Verification items for the finished model (mm, model axes). Face numbers are marked on the shaded views. Give positions to 0.01 mm unless a question says otherwise; leave off trailing zeros. Write each loop counter-clockwise with the first axis right and the second up, starting at its lowest first coordinate (ties: lowest second). Pieces come first, ordered by that corner, then holes.
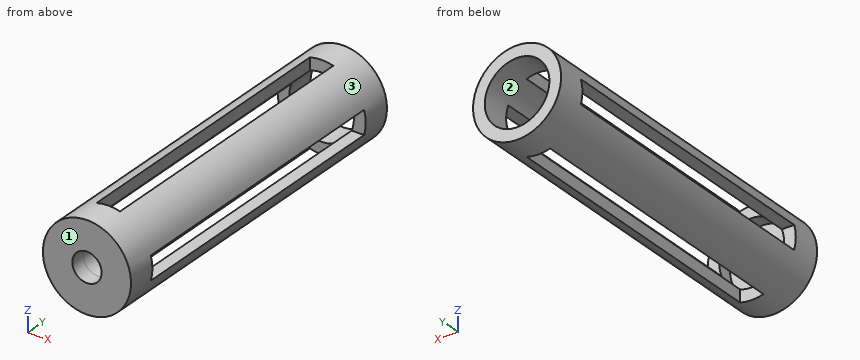
from build123d import *

# Parameters (mm, degrees)
SKETCH1_R               = 19.05
SKETCH1_R_2             = 13.97
BOSS_EXTRUDE1_DEPTH     = 152.4
SKETCH2_R               = 13.97
BOSS_EXTRUDE2_DEPTH     = 6.35
SKETCH3_R               = 2.2479
CUT_EXTRUDE1_DEPTH      = 3.54
CUT_EXTRUDE1_DEPTH_BACK = 36.56
SKETCH5_W               = 10.16
SKETCH5_H               = 127
CUT_EXTRUDE5_DEPTH      = 20.0500001
CUT_EXTRUDE5_DEPTH_BACK = 20.0500001
SKETCH8_W               = 10.16
SKETCH8_H               = 127
CUT_EXTRUDE6_DEPTH      = 20.050000101
CUT_EXTRUDE6_DEPTH_BACK = 20.050000101
SKETCH7_R               = 6.35
CUT_EXTRUDE4_DEPTH      = 7.35
SKETCH9_R               = 8.89
SKETCH9_R_2             = 6.35
BOSS_EXTRUDE3_DEPTH     = 19.05
SKETCH10_R              = 8.89
SKETCH10_R_2            = 5.08
BOSS_EXTRUDE4_DEPTH     = 5.08


with BuildPart() as part:
    # Sketch1 → Boss-Extrude1 (new body)
    with BuildSketch(Plane(origin=(0, 0, 0), x_dir=(1, 0, 0), z_dir=(0, 1, 0))):
        Circle(SKETCH1_R)
        Circle(SKETCH1_R_2, mode=Mode.SUBTRACT)
    extrude(amount=BOSS_EXTRUDE1_DEPTH)

    # Sketch2 → Boss-Extrude2 (add)
    with BuildSketch(Plane.XZ):
        Circle(SKETCH2_R)
    extrude(amount=-BOSS_EXTRUDE2_DEPTH)

    # Sketch3 → Cut-Extrude1 (cut, two sides)
    with BuildSketch(Plane.XY.offset(16.51)) as cut_extrude1_sk:
        with Locations((0, 101.6)):
            Circle(SKETCH3_R)
    extrude(amount=CUT_EXTRUDE1_DEPTH, mode=Mode.SUBTRACT)
    extrude(cut_extrude1_sk.sketch, amount=-CUT_EXTRUDE1_DEPTH_BACK, mode=Mode.SUBTRACT)

    # Sketch5 → Cut-Extrude5 (cut, two sides)
    with BuildSketch(Plane(origin=(0, 0, 0), x_dir=(0, 0, -1), z_dir=(1, 0, 0))) as cut_extrude5_sk:
        with Locations((0, 76.2)):
            Rectangle(SKETCH5_W, SKETCH5_H)
    extrude(amount=CUT_EXTRUDE5_DEPTH, mode=Mode.SUBTRACT)
    extrude(cut_extrude5_sk.sketch, amount=-CUT_EXTRUDE5_DEPTH_BACK, mode=Mode.SUBTRACT)

    # Sketch8 → Cut-Extrude6 (cut, two sides)
    with BuildSketch(Plane.XY) as cut_extrude6_sk:
        with Locations((0, 76.2)):
            Rectangle(SKETCH8_W, SKETCH8_H)
    extrude(amount=CUT_EXTRUDE6_DEPTH, mode=Mode.SUBTRACT)
    extrude(cut_extrude6_sk.sketch, amount=-CUT_EXTRUDE6_DEPTH_BACK, mode=Mode.SUBTRACT)

    # Sketch7 → Cut-Extrude4 (cut, through all)
    with BuildSketch(Plane(origin=(0, 6.35, 0), x_dir=(1, 0, 0), z_dir=(0, 1, 0))):
        Circle(SKETCH7_R)
    extrude(amount=-CUT_EXTRUDE4_DEPTH, mode=Mode.SUBTRACT)

    # Sketch9 → Boss-Extrude3 (add)
    with BuildSketch(Plane(origin=(0, 6.35, 0), x_dir=(1, 0, 0), z_dir=(0, 1, 0))):
        Circle(SKETCH9_R)
        Circle(SKETCH9_R_2, mode=Mode.SUBTRACT)
    extrude(amount=BOSS_EXTRUDE3_DEPTH)

    # Sketch10 → Boss-Extrude4 (add)
    with BuildSketch(Plane(origin=(0, 25.4, 0), x_dir=(1, 0, 0), z_dir=(0, 1, 0))):
        Circle(SKETCH10_R)
        Circle(SKETCH10_R_2, mode=Mode.SUBTRACT)
    extrude(amount=BOSS_EXTRUDE4_DEPTH)


solid = part.part
Item 1: Scan lines: line 1 along Y through (x, z) = (2, 16); line 2 along X through (y, z) = (20.5, 0). Record each from-to range of solid material in increasing order.
Answer key:
line 1: y = 0 to 12.7, 139.7 to 152.4
line 2: x = -8.89 to -6.35, 6.35 to 8.89
Item 2: Release check for a two-part mould opening along Z. For the marked faces 1, 2 and 3 record: released by +Z, released by -Z, zero draft, split by the parting line, or undercut.
Answer key:
face 1: zero draft
face 2: undercut
face 3: split by the parting line
Item 3: Depth check by flat-ended pin: pin 1 (3 mm diameter, centred on x = -16.5, z = 2.5, fed in from -Y); pin 2 (4.5 mm diameter, centred on x = 14.5, y = 55, fed in from -Z); pin 3 (1.6 mm diameter, centred on x = -15.5, y = 106.5, fed in from -Z); pin 4 (3 mm diameter, centred on x = -7.5, y = 117, fed in from +Z). Enter the tip coordinate at first touch or a pass-through.
Answer key:
pin 1: stops at y = 0
pin 2: stops at z = -14.59
pin 3: stops at z = -12.12
pin 4: stops at z = 18.08
Item 4: Sectioned sample at C-C on x = 0. Record the cut outline in (y, z).
Answer key:
outline: (0, -19.05) - (12.7, -19.05) - (12.7, -13.97) - (6.35, -13.97) - (6.35, -8.89) - (30.48, -8.89) - (30.48, -5.08) - (25.4, -5.08) - (25.4, -6.35) - (0, -6.35) - close; (0, 6.35) - (25.4, 6.35) - (25.4, 5.08) - (30.48, 5.08) - (30.48, 8.89) - (6.35, 8.89) - (6.35, 13.97) - (12.7, 13.97) - (12.7, 19.05) - (0, 19.05) - close; (139.7, -19.05) - (152.4, -19.05) - (152.4, -13.97) - (139.7, -13.97) - close; (139.7, 13.97) - (152.4, 13.97) - (152.4, 19.05) - (139.7, 19.05) - close
Item 5: Sectioned sample at D-D on z = -15.5. Record the cut outline in (x, y), then the cut area to 3 significant figures.
Answer key:
outline: (-11.07, 0) - (11.07, 0) - (11.07, 152.4) - (-11.07, 152.4) - close; hole (-5.08, 12.7) - (5.08, 12.7) - (5.08, 139.7) - (-5.08, 139.7) - close
area: 2,090 mm2
Item 6: Sectioned sample at A-A on z = 0. Record the cut outline in (x, y).
Answer key:
outline: (-19.05, 0) - (-6.35, 0) - (-6.35, 25.4) - (-5.08, 25.4) - (-5.08, 30.48) - (-8.89, 30.48) - (-8.89, 6.35) - (-13.97, 6.35) - (-13.97, 12.7) - (-19.05, 12.7) - close; (-19.05, 139.7) - (-13.97, 139.7) - (-13.97, 152.4) - (-19.05, 152.4) - close; (5.08, 25.4) - (6.35, 25.4) - (6.35, 0) - (19.05, 0) - (19.05, 12.7) - (13.97, 12.7) - (13.97, 6.35) - (8.89, 6.35) - (8.89, 30.48) - (5.08, 30.48) - close; (13.97, 139.7) - (19.05, 139.7) - (19.05, 152.4) - (13.97, 152.4) - close
Item 7: Sectioned sample at B-B on y = 125. Record the cut outline in (x, z), then the cut area to 3 significant figures.
Answer key:
outline: (-18.36, -5.08) arc R19.05 ccw to (-5.08, -18.36) - (-5.08, -13.01) arc R13.97 cw to (-13.01, -5.08) - close; (-18.36, 5.08) - (-13.01, 5.08) arc R13.97 cw to (-5.08, 13.01) - (-5.08, 18.36) arc R19.05 ccw to start; (5.08, -18.36) arc R19.05 ccw to (18.36, -5.08) - (13.01, -5.08) arc R13.97 cw to (5.08, -13.01) - close; (5.08, 13.01) arc R13.97 cw to (13.01, 5.08) - (18.36, 5.08) arc R19.05 ccw to (5.08, 18.36) - close
area: 317 mm2
